For this review, take the finished solid that the model builds, in its own axes (mm). Face numbers are marked on the shaded views. A direction names the side the tool comes from. Coordinates: 2 decimals unless noted, no trailing zeros. Write each loop counter-clockwise with the first axis right and the second up, starting at its lowest first coordinate (ties: lowest second). Pieces come first, ordered by that corner, then holes.
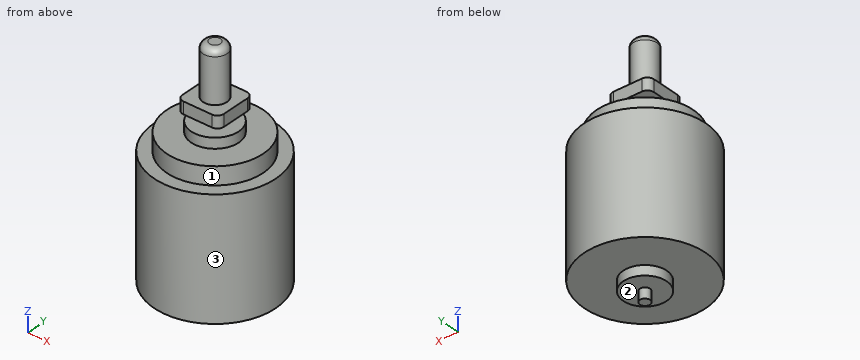
```python
from build123d import *

# Parameters (mm, degrees)
F2_W     = 8.1026
F2_H     = 8.1026
F2_R     = 2.3368
F3_DEPTH = 2.3368
F4_R     = 1.27
F5_R     = 1.27


with BuildPart() as f1:
    # F0 (on Front) → F1 (revolve)
    with BuildSketch(Plane.XZ):
        Polygon((11.8491, -23.3426), (11.8491, 0), (9.398, 0), (9.398, 3.4544), (4.635883, 3.4544), (4.635883, 5.461), (1.016, 5.461), (1.016, 7.4676), (2.3368, 7.4676), (2.3368, 19.7612), (0, 19.7612), (0, -27.2542), (1.0033, -27.2542), (1.0033, -25.2476), (4.2291, -25.2476), (4.2291, -23.3426), align=None)
    revolve(axis=Axis((0, 0, -3.7465), (0, 0, -1)))

    # F2 (on face) → F3 (join)
    with BuildSketch(Plane(origin=(0, 0, 7.4676), x_dir=(1, 0, 0), z_dir=(0, 0, -1))):
        Rectangle(F2_W, F2_H)
        Circle(F2_R, mode=Mode.SUBTRACT)
    extrude(amount=-F3_DEPTH)

    # F4
    f4_edges = [f1.edges().sort_by_distance(p)[0] for p in [
        (4.0513, -4.0513, 8.636),
        (-4.0513, -4.0513, 8.636),
        (-4.0513, 4.0513, 8.636),
        (4.0513, 4.0513, 8.636),
    ]]
    fillet(f4_edges, radius=F4_R)

    # F5
    f5_edges = [f1.edges().sort_by_distance(p)[0] for p in [
        (-2.3368, 0, 19.7612),
    ]]
    fillet(f5_edges, radius=F5_R)


solid = f1.part
```
Q1. Add section D-D (y = -8.75). State the section outline as (x, z) points.
Ans:
outline: (-7.99, -23.34) - (7.99, -23.34) - (7.99, 0) - (3.43, 0) - (3.43, 3.45) - (-3.43, 3.45) - (-3.43, 0) - (-7.99, 0) - close
Q2. For probe 1 along Z at (x, y) = (3.5, -3.5); probe 2 along Z at (x, y) = (-2, -3.25); probe 3 along Z at (x, y) = (4.25, -9.5), list the stretches that pass through material, from the lowest coordinate up.
Ans:
probe 1: z = -23.34 to 3.45, 7.47 to 9.8
probe 2: z = -25.25 to 5.46, 7.47 to 9.8
probe 3: z = -23.34 to 0
Q3. Add section C-C (z = 0.5). State the section outline as (x, y) points.
Ans:
outline: circle Ø18.8 at (0, 0)
Q4. Clearance check with flat-ended pins moving along their axes: pin 1 Ø8 at (x, y) = (-8.5, 7) entering from +Z; pin 2 Ø2 at (y, z) = (-2.5, -10.5) entering from -X; pin 3 Ø2.5 at (y, z) = (1, 8) entering from +X. State where each tip first meets the part, or that it passes through.
Ans:
pin 1: stops at z = 3.45
pin 2: stops at x = -11.75
pin 3: stops at x = 4.05
Q5. Tool access review of the marked faces 1, 2 and 3: name each direction out of +Z, -Z, +X, -X, +Y, -Y from which nothing blocks a thin tool from reaching the whole face with its end or side.
Ans:
face 1: +Z
face 2: -Z
face 3: +Z, -Z
Q6. Add section B-B (x = -7.75). State the section outline as (y, z) points.
Ans:
outline: (-8.96, -23.34) - (8.96, -23.34) - (8.96, 0) - (5.32, 0) - (5.32, 3.45) - (-5.32, 3.45) - (-5.32, 0) - (-8.96, 0) - close
Q7. Add section A-A (x = -3.25). State the section outline as (y, z) points.
Ans:
outline: (-11.39, -23.34) - (-2.71, -23.34) - (-2.71, -25.25) - (2.71, -25.25) - (2.71, -23.34) - (11.39, -23.34) - (11.39, 0) - (8.82, 0) - (8.82, 3.45) - (3.31, 3.45) - (3.31, 5.46) - (-3.31, 5.46) - (-3.31, 3.45) - (-8.82, 3.45) - (-8.82, 0) - (-11.39, 0) - close; (-3.96, 7.47) - (3.96, 7.47) - (3.96, 9.8) - (-3.96, 9.8) - close
